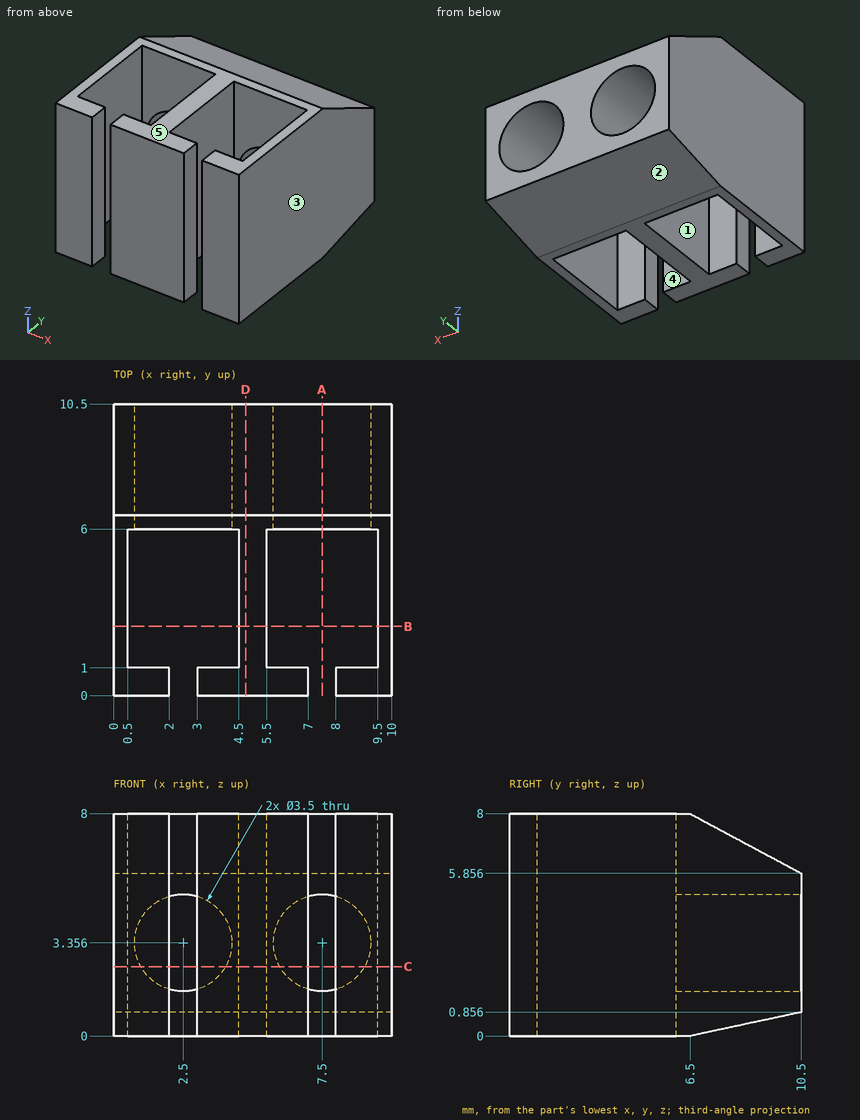
Answer from the drawing. Dimensions are ordinates in mm from the lowest x, y and z of the part. A direction names the side the tool comes from. Give positions to 0.01 mm unless a question says otherwise; leave off trailing zeros. Loops run counter-clockwise (first coordinate to the right, second up) from the corner with the lowest first, then second, coordinate; pieces in that order, holes last.
Item 1: Each of these flat-tipped pins is pushed along its axis until it touches: pin 1 Ø0.5 at (y, z) = (0.5, 5) entering from -X; pin 2 Ø4 at (x, y) = (3, 9) entering from -Z. Where does it stop, or does it pass through?
Item 2: The part is cut by section B-B (y = 2.5). Write down the section's boundary in (x, z), and give its area (3 significant figures).
Item 3: The mould has two halves that part along X. Classify the marked faces 1, 2 and 3: released by +X, released by -X, zero draft, split by the parting line, or undercut.
Item 4: Find the intervals of material crossed by line 1 along X through (y, z) = (4.5, 3.75); line 2 along X through (y, z) = (0.75, 6.5); line 3 along Y through (x, z) = (1.25, 1), in increasing order.
Item 5: For the marked faces 4 and 5, determine the directions among +Z, -Z, +X, -X, +Y, -Y from which every point of the face is accessible in a straight line to the end or side of a thin tool.
Item 6: The part is cut by section D-D (x = 4.75). Write down the section's boundary in (y, z), and give its area (3 significant figures).
Item 7: The part is cut by section C-C (z = 2.5). Write down the section's boundary in (x, y).
Item 8: The part is cut by section A-A (x = 7.5). Write down the section's boundary in (y, z).
Taken from the geometry:
1. pin 1: stops at x = 0
1. pin 2: stops at z = 0.11
2. outline: (0, 0) - (0.5, 0) - (0.5, 8) - (0, 8) - close; (4.5, 0) - (5.5, 0) - (5.5, 8) - (4.5, 8) - close; (9.5, 0) - (10, 0) - (10, 8) - (9.5, 8) - close
2. area: 16.0 mm2
3. face 1: undercut
3. face 2: zero draft
3. face 3: released by +X
4. line 1: x = 0 to 0.5, 4.5 to 5.5, 9.5 to 10
4. line 2: x = 0 to 2, 3 to 7, 8 to 10
4. line 3: y = 0 to 1, 6 to 10.5
5. face 4: +Z, -Z
5. face 5: +Z, +X, -X, +Y, -Y
6. outline: (0, 0) - (6.5, 0) - (10.5, 0.86) - (10.5, 5.86) - (6.5, 8) - (0, 8) - close
6. area: 78.0 mm2
7. outline: (0, 0) - (2, 0) - (2, 1) - (0.5, 1) - (0.5, 6) - (0.97, 6) - (0.97, 10.5) - (0, 10.5) - close; (3, 0) - (7, 0) - (7, 1) - (5.5, 1) - (5.5, 6) - (5.97, 6) - (5.97, 10.5) - (4.03, 10.5) - (4.03, 6) - (4.5, 6) - (4.5, 1) - (3, 1) - close; (8, 0) - (10, 0) - (10, 10.5) - (9.03, 10.5) - (9.03, 6) - (9.5, 6) - (9.5, 1) - (8, 1) - close
8. outline: (6, 0) - (6.5, 0) - (10.5, 0.86) - (10.5, 1.61) - (6, 1.61) - close; (6, 5.11) - (10.5, 5.11) - (10.5, 5.86) - (6.5, 8) - (6, 8) - close
